Input: part model. Units: mm. Frame: model coordinates. A direction names the side the tool comes from. Give positions to 0.01 mm unless a question says otherwise; leave off trailing zeros. Write each loop counter-clockwise with the first axis right and the second up, starting at its lowest first coordinate (ties: lowest second). Pieces come first, ordered by that corner, then holes.
```python
from build123d import *

# Parameters (mm, degrees)
SKETCH1_R           = 4.7625
BOSS_EXTRUDE1_DEPTH = 15
CUT_EXTRUDE1_DEPTH  = 16


with BuildPart() as part:
    # Sketch1 → Boss-Extrude1 (new body)
    with BuildSketch(Plane(origin=(0, 0, 0), x_dir=(1, 0, 0), z_dir=(0, 1, 0))):
        with BuildLine():
            Line((-16.25, 28.145825623), (-5, 8.660254038))
            ThreePointArc((-5, 8.660254038), (0, 10), (5, 8.660254038))
            Line((5, 8.660254038), (16.25, 28.145825623))
            ThreePointArc((16.25, 28.145825623), (0, -32.5), (-16.25, 28.145825623))
        make_face()
        Circle(SKETCH1_R, mode=Mode.SUBTRACT)
    extrude(amount=BOSS_EXTRUDE1_DEPTH)

    # Sketch4 → Cut-Extrude1 (cut, through all)
    with BuildSketch(Plane(origin=(0, 15, 0), x_dir=(1, 0, 0), z_dir=(0, 1, 0))):
        with BuildLine():
            Line((11.490666647, -9.641814145), (45.503789868, 30.893447649))
            ThreePointArc((45.503789868, 30.893447649), (34.992750198, -42.432386612), (-38.992939572, -38.788537785))
            Line((-38.992939572, -38.788537785), (11.490666647, -9.641814145))
        make_face()
    extrude(amount=-CUT_EXTRUDE1_DEPTH, mode=Mode.SUBTRACT)


solid = part.part
```
Item 1: Section D-D (x = -10.5). Return loops of the section in (y, z), and give its area (3 significant figures).
Item 2: Mould query, pull axis X, two halves, no side actions, for faces 3 (the cylindrical face through (-3.78, 7.4, 2.9)), 4 (the flat face through (10.55, 7.4, -18.27)), 5 (the cylindrical face through (-32.49, 7.4, -0.76)), 6 (the flat face through (-8, 15, -1)). Classes: +X half, -X half, draft (parallel to the pull), parting line (faces both ways), or undercut.
Item 3: Pin query (flat end, axial travel): pin 1 (5 mm diameter, centred on y = 10.5, z = -13, fed in from -X); pin 2 (1.5 mm diameter, centred on y = 5.5, z = -8, fed in from +X); pin 3 (4 mm diameter, centred on x = -13, y = 3, fed in from +Z). Return the tip coordinate at first contact, or that it passes through.
Item 4: Ray query, line 1 (X direction, y = 5, z = 0); line 2 (Z direction, x = -0.5, y = 6.5); line 3 (Z direction, x = 0, y = 6.25). Return the intervals inside material, ascending.
Item 5: Section B-B (x = 2). Return loops of the section in (y, z).
Item 6: Section C-C (z = 0). Return loops of the section in (x, y).
Item 7: Set-up query: faces 1 (the flat face through (-10.704, 7.395, -18.539)), 2 (the flat face through (20.63, 7.6, -1.25)). Return all of +Z, -Z, +X, -X, +Y, -Y with unobstructed straight access to the full face (end or side cutting, diameter ignored); none if empty.
Solved:
1. outline: (0, -18.19) - (15, -18.19) - (15, 22.34) - (0, 22.34) - close
1. area: 608 mm2
2. face 3: undercut
2. face 4: undercut
2. face 5: -X half
2. face 6: draft
3. pin 1: stops at x = -30.76
3. pin 2: stops at x = 26.92
3. pin 3: stops at z = 24.94
4. line 1: x = -32.5 to -4.76, 4.76 to 19.58
4. line 2: z = -9.99 to -4.74, 4.74 to 16.56
4. line 3: z = -10 to -4.76, 4.76 to 16.28
5. outline: (0, -9.8) - (15, -9.8) - (15, -4.32) - (0, -4.32) - close; (0, 4.32) - (15, 4.32) - (15, 15.12) - (0, 15.12) - close
6. outline: (-32.5, 0) - (-4.76, 0) - (-4.76, 15) - (-32.5, 15) - close; (4.76, 0) - (19.58, 0) - (19.58, 15) - (4.76, 15) - close
7. face 1: -Z, +Y, -Y
7. face 2: +Z, +X, +Y, -Y
